Geometry check sheet. Reference: the model listing, model coordinates, mm. Face numbers are marked on the shaded views. A direction names the side the tool comes from. Round coordinates to 2 decimals unless told otherwise and drop trailing zeros. Write each loop counter-clockwise with the first axis right and the second up, starting at its lowest first coordinate (ties: lowest second). Pieces come first, ordered by that corner, then holes. Notation, with made-up numbers: (65, -7.75) -> (71, -7.75) arc R13 ccw to (71, 8.25) -> close; hole circle Ø5 at (-28.75, -37.5). An arc over 180 degrees is marked (long way). Use a Markdown table: item, result.
```python
from build123d import *

# Parameters (mm, degrees)
F1_DEPTH      = 6
F3_DEPTH      = 9
F3_DEPTH_BACK = 9
F4_R          = 6.25
F5_DEPTH      = 25
F6_D          = 3
F7_R          = 5


with BuildPart() as f1:
    # F0 (on Top) → F1 (new body)
    with BuildSketch(Plane.XY):
        with BuildLine():
            Line((6.25, -12.4998748011), (12.9519546771, -12.4998748011))
            ThreePointArc((12.9519546771, -12.4998748011), (0, 18), (-12.9519546771, -12.4998748011))
            Line((-12.9519546771, -12.4998748011), (-6.25, -12.4998748011))
            Line((-6.25, -12.4998748011), (-6.25, 0))
            ThreePointArc((-6.25, 0), (0, 6.25), (6.25, 0))
            Line((6.25, 0), (6.25, -12.4998748011))
        make_face()
    extrude(amount=F1_DEPTH)

    # F2 (on Right) → F3 (join, two sides)
    with BuildSketch(Plane.YZ) as f3_sk:
        Polygon((11.0055337464, 0), (22.9271929711, 0), (25.7638388276, 16), (43.7638388276, 16), (43.7638388276, 19.5), (21.7638388276, 19.5), (18.7638388276, 6), (11.0055337464, 6), align=None)
    extrude(amount=F3_DEPTH)
    extrude(f3_sk.sketch, amount=-F3_DEPTH_BACK)

    # F4 (on face) → F5 (cut)
    with BuildSketch(Plane(origin=(0, 0, 16), x_dir=(1, 0, 0), z_dir=(0, 0, -1))):
        with Locations((0, -34.7638388276)):
            Circle(F4_R)
    extrude(amount=-F5_DEPTH, mode=Mode.SUBTRACT)

    # F6 (through all)
    with Locations(Plane(origin=(0, 0, 0), x_dir=(1, 0, 0), z_dir=(0, 0, -1))):
        with Locations((10.7972361083, -6.2983880813), (10.8531821354, 6.2014867198), (-0.0559460271, -12.4998748011), (-10.8531821354, -6.2014867198), (-10.7972361083, 6.2983880813)):
            Hole(F6_D / 2)

    # F7
    f7_edges = [f1.edges().sort_by_distance(p)[0] for p in [
        (0, 18.763839, 6),
        (0, 21.763839, 19.5),
        (0, 22.927193, 0),
        (-9, 43.763839, 17.75),
        (9, 43.763839, 17.75),
    ]]
    fillet(f7_edges, radius=F7_R)


solid = f1.part
```
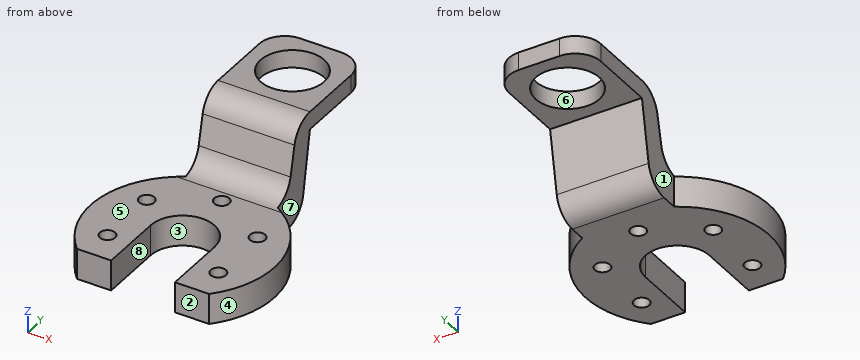
(1) Thickness scan on line 1 (X direction, y = 22, z = 7.5); line 2 (Z direction, x = -14.5, y = 10.5); line 3 (Y direction, x = 10, z = 5.5). Record the ranges inside material, lowest first.
A:
| item | result |
|---|---|
| line 1 | x = -9 to 9 |
| line 2 | z = 0 to 6 |
| line 3 | y = -12.5 to -7.44, -4.97 to 5.03, 7.57 to 14.97 |
(2) Section check C-C on z = 13. Record the cut outline in (x, y), plus the area to 3 significant figures.
A:
| item | result |
|---|---|
| outline | (-9, 20.32) -> (9, 20.32) -> (9, 25.23) -> (-9, 25.23) -> close |
| area | 88.4 mm2 |
(3) Section check A-A on x = 0. Record the cut outline in (y, z), plus the area to 3 significant figures.
A:
| item | result |
|---|---|
| outline | (6.25, 0) -> (11, 0) -> (11, 6) -> (6.25, 6) -> close; (14, 0) -> (18.74, 0) arc R5 ccw to (23.66, 4.13) -> (25.76, 16) -> (28.51, 16) -> (28.51, 19.5) -> (25.77, 19.5) arc R5 ccw to (20.89, 15.58) -> (19.63, 9.92) arc R5 cw to (14.75, 6) -> (14, 6) -> close; (41.01, 16) -> (43.76, 16) -> (43.76, 19.5) -> (41.01, 19.5) -> close |
| area | 166 mm2 |
(4) Section check D-D on x = 15.5. Record the cut outline in (y, z), plus the area to 3 significant figures.
A:
| item | result |
|---|---|
| outline | (-9.15, 0) -> (9.15, 0) -> (9.15, 6) -> (-9.15, 6) -> close |
| area | 110 mm2 |
(5) Gauge pin test, flat ends, axial feed: pin 1 Ø3 at (y, z) = (-6, 2) entering from -X; pin 2 Ø3 at (y, z) = (5.5, 8.5) entering from +X; pin 3 Ø9 at (x, y) = (-2, 36.5) entering from -Z; pin 4 Ø1.8 at (y, z) = (-4.5, 2.5) entering from +X. Record the tip position at first contact, or that the pin passes through.
A:
| item | result |
|---|---|
| pin 1 | stops at x = -17.43 |
| pin 2 | passes through |
| pin 3 | stops at z = 16 |
| pin 4 | stops at x = 17.64 |
(6) Release check for a two-part mould opening along X. For the marked faces 1, 2, 3 and 4 record: +X half, -X half, draft (parallel to the pull), parting line (faces both ways), or undercut.
A:
| item | result |
|---|---|
| face 1 | -X half |
| face 2 | draft |
| face 3 | undercut |
| face 4 | +X half |
(7) Section check B-B on y = 3.5. Record the cut outline in (x, z).
A:
| item | result |
|---|---|
| outline | (-17.66, 0) -> (-5.18, 0) -> (-5.18, 6) -> (-17.66, 6) -> close; (5.18, 0) -> (17.66, 0) -> (17.66, 6) -> (5.18, 6) -> close |
(8) Access from +Z, -Z, +X, -X, +Y, -Y to the whole of each face (thin tool, end or side, straight path). Record for the marked faces 5, 6, 7 and 8.
A:
| item | result |
|---|---|
| face 5 | +Z, +X, -X, -Y |
| face 6 | +Z, -Z |
| face 7 | +Z, -Z, +X, +Y |
| face 8 | +Z, -Z, -Y |
